Check sheet for the modelled part. Datum: model origin and axes. Units: mm. Round coordinates to 2 decimals unless told otherwise and drop trailing zeros. Write each loop counter-clockwise with the first axis right and the second up, starting at its lowest first coordinate (ties: lowest second). Pieces come first, ordered by that corner, then holes. Notation, with made-up numbers: M -39.5,-3.75 L 7.5,-3.75 A29 cw 7.5,29.25 Z; hole C 89,89.5 d1. An arc over 180 degrees is marked long. Put each result on its own line as item: value.
Autodesk Inventor part; units mm, degrees
ref_plane "YZ Plane" through (0, 0, 0) normal (1, 0, 0) x (0, 1, 0)
ref_plane "XZ Plane" through (0, 0, 0) normal (0, 1, 0) x (-1, 0, 0)
ref_plane "XY Plane" through (0, 0, 0) normal (0, 0, 1) x (1, 0, 0)
sketch "Náčrt1" plane through (0, 0, 0) normal (0, 1, 0) x (-1, 0, 0)
  line L0 (160, 175) -> (-160, 175)
  line L1 (-160, 175) -> (-160, -175)
  line L2 (-160, -175) -> (160, -175)
  line L3 (160, -175) -> (160, 175)
  line L4 (160, 175) -> (-160, -175) construction
  line L5 (-160, 175) -> (160, -175) construction
  point P0 (0, 0)
  dimension "d0" = 320
  dimension "d1" = 350
extrude "Vysunutí1" add sketch "Náčrt1" along normal blind 10
sketch "Náčrt3" plane through (0, 0, 0) normal (0, -1, 0) x (1, 0, 0)
  line L0 (160, -175) -> (-160, -175)
  line L1 (160, 175) -> (160, -175)
  point P0 (0, 0)
  point P1 (60, -95)
  point P2 (60, 25)
  point P3 (-60, 25)
  point P4 (-60, -95)
  dimension "d14" = 120
  dimension "d15" = 120
  dimension "d16" = 80
  dimension "d17" = 100
hole "Díra1" at (60, 0, -95) at (60, 0, 25) at (-60, 0, 25) at (-60, 0, -95) direction (0, 1, 0) diameter 10 end through all
sketch "Náčrt4" plane through (0, 0, 0) normal (0, -1, 0) x (1, 0, 0)
  line L0 (-160, 175) -> (160, 175)
  line L1 (-160, -175) -> (-160, 175)
  line L2 (160, 175) -> (160, -175)
  line L3 (160, -175) -> (-160, -175)
  point P0 (0, 0)
  point P1 (-140, 155)
  point P2 (140, 155)
  point P3 (-140, -155)
  point P4 (140, -155)
  dimension "d25" = 20
  dimension "d26" = 20
  dimension "d27" = 20
  dimension "d28" = 20
hole "Díra2" at (-140, 0, 155) at (140, 0, 155) at (-140, 0, -155) at (140, 0, -155) direction (0, 1, 0) diameter 2 depth 9
properties part number "deska" material "Dřevo (Bříza)"
1. Release check for a two-part mould opening along Z. For faces 1 (the flat face through (2, 5, -175)), 2 (the cylindrical face through (-64, 5, -98)), 3 (the cylindrical face through (56, 5, -98)), 4 (the flat face through (160, 5, 2)) record: +Z half, -Z half, draft (parallel to the pull), parting line (faces both ways), or undercut.
Computed values:
face 1: -Z half
face 2: undercut
face 3: undercut
face 4: draft
2. Scan lines: probe 1 along Z at (x, y) = (-60, 2); probe 2 along X at (y, z) = (5.25, -95); probe 3 along Z at (x, y) = (140, 3.5). Record each from-to range of solid material in increasing order.
Computed values:
probe 1: z = -175 to -100, -90 to 20, 30 to 175
probe 2: x = -160 to -65, -55 to 55, 65 to 160
probe 3: z = -175 to -156, -154 to 154, 156 to 175
3. Cross-section at A-A (z = 25). Enter the section's corners in (x, y), then the cut area to 3 significant figures.
Computed values:
outline: M -160,0 L -65,0 L -65,10 L -160,10 Z; M -55,0 L 55,0 L 55,10 L -55,10 Z; M 65,0 L 160,0 L 160,10 L 65,10 Z
area: 3,000 mm2
4. Cross-section at B-B (x = 60). Enter the section's corners in (y, z), then the cut area to 3 significant figures.
Computed values:
outline: M 0,-175 L 10,-175 L 10,-100 L 0,-100 Z; M 0,-90 L 10,-90 L 10,20 L 0,20 Z; M 0,30 L 10,30 L 10,175 L 0,175 Z
area: 3,300 mm2
5. Depth check by flat-ended pin: pin 1 Ø1.8 at (x, z) = (140, 155) entering from -Y; pin 2 Ø6 at (x, z) = (60, -95) entering from +Y. Enter the tip coordinate at first touch or a pass-through.
Computed values:
pin 1: stops at y = 9
pin 2: passes through
